Read the model definition and answer for the solid it produces. Units are mm, in the model's axes. Coordinates: 2 decimals unless noted, no trailing zeros. Write each loop counter-clockwise with the first axis right and the second up, starting at its lowest first coordinate (ties: lowest second). Pieces come first, ordered by that corner, then holes. Notation, with made-up numbers: (22, 53.5) -> (28, 53.5) arc R11 ccw to (28, 64.5) -> close; hole circle Ø10 at (19, -32). An arc over 180 degrees is marked (long way). Answer as a JSON object with one key per item and string values. Group by question number.
(1) Find section A-A (y = -19.15). Give the vertices of the cut face in (x, z) (3 decimals), then the cut area to 3 significant figures.
(2) Straight lines are drawn through the part: L1, parallel to X at y = -19.15, z = 1.5 (3 decimals); L2, parallel to Y at x = -14.5, z = 2.9; L3, parallel to X at y = -18, z = 1.85. For each, find the intervals that lie inside material, in ascending order.
(3) Find section D-D (x = -10.15). Give the vertices of the cut face in (y, z) (3 decimals), then the cut area to 3 significant figures.
(4) For a pull along Y with two mould halves and no side action, classify faces 1 (the face through (16.475, -7.375, 1.362)), 2 (the face through (-21.15, 0, 2)), 3 (the face through (0, 28, 2)), 4 (the face through (0, -28, 2)) as +Y half, -Y half, draft (parallel to the pull), parting line (faces both ways), or undercut.
(5) Find section C-C (y = 13). Give the vertices of the cut face in (x, z) (3 decimals), then the cut area to 3 significant figures.
(6) Find section B-B (x = 0). Give the vertices of the cut face in (y, z) (3 decimals), then the cut area to 3 significant figures.
Autodesk Inventor part; units mm, degrees
ref_plane "YZ Plane" through (0, 0, 0) normal (1, 0, 0) x (0, 1, 0)
ref_plane "XZ Plane" through (0, 0, 0) normal (0, 1, 0) x (-1, 0, 0)
ref_plane "XY Plane" through (0, 0, 0) normal (0, 0, 1) x (1, 0, 0)
sketch "Sketch1" plane through (0, 0, 0) normal (0, 0, 1) x (1, 0, 0)
  line L0 (-21.15, 28) -> (21.15, 28)
  line L1 (21.15, 28) -> (21.15, -28)
  line L2 (21.15, -28) -> (-21.15, -28)
  line L3 (-21.15, -28) -> (-21.15, 28)
  point P0 (0, 0)
  dimension "d0" = 56
  dimension "d1" = 42.3
  dimension "d2" = 21.15
  dimension "d3" = 28
  dimension "d44" = 21.15
extrude "Extrusion1" add sketch "Sketch1" along normal blind 3.175
sketch "Sketch2" plane through (0, 0, 3.175) normal (0, 0, 1) x (1, 0, 0)
  circle A0 centre (-15.499, 22.359) radius 1.5875
  circle A1 centre (15.499, 22.359) radius 1.5875
  line L0 (21.15, 28) -> (-21.15, 28)
  line L1 (-21.15, 28) -> (-21.15, -28)
  line L2 (21.15, -28) -> (21.15, 28)
  circle A2 centre (-15.509, -8.635) radius 1.5875
  circle A3 centre (15.509, -8.635) radius 1.5875
  point P0 (0, 0)
  dimension "d6" = 3.175
  dimension "d7" = 5.641
  dimension "d8" = 5.641
  dimension "d9" = 5.651
  dimension "d10" = 5.651
  dimension "d11" = 3.175
  dimension "d45" = 3.175
  dimension "d46" = 3.175
  dimension "d47" = 5.641
  dimension "d48" = 5.641
  dimension "d49" = 36.635
  dimension "d50" = 36.635
hole "Hole1" at (-15.499, 22.359, 3.175) at (15.499, 22.359, 3.175) at (-15.509, -8.635, 3.175) at (15.509, -8.635, 3.175) direction (0, 0, -1) diameter 3.175 end through all countersink diameter 4 countersink angle 90
sketch "Sketch3" plane through (0, 0, 3.175) normal (0, 0, 1) x (1, 0, 0)
  circle A0 centre (-10.15, -19.15) radius 3.175
  circle A1 centre (10.15, -19.15) radius 3.175
  line L0 (-21.15, -28) -> (21.15, -28)
  line L1 (21.15, -28) -> (21.15, 28)
  line L2 (-21.15, 28) -> (-21.15, -28)
  line L3 (21.15, 28) -> (-21.15, 28)
  point P0 (0, 0)
  dimension "d19" = 6.35
  dimension "d20" = 6.35
  dimension "d22" = 11
  dimension "d23" = 11
  dimension "d25" = 47.15
  dimension "d26" = 47.15
hole "Hole2" at (-10.15, -19.15, 3.175) at (10.15, -19.15, 3.175) direction (0, 0, -1) diameter 6.35 end through all
sketch "Sketch5" plane through (0, 0, 0) normal (0, 0, -1) x (-1, 0, 0)
  circle A0 centre (0, 6.756) radius 11.5
  line L0 (21.15, 28) -> (-21.15, 28)
  line L1 (21.15, -28) -> (21.15, 28)
  point P0 (0, 0)
  dimension "d39" = 23
  dimension "d40" = 21.244
  dimension "d41" = 21.15
extrude "Extrusion3" cut sketch "Sketch5" against normal through all
properties part number "MOTOR MOUNT"
Results below:
{
 "1": {"outline": "(-21.15, 0) -> (-13.325, 0) -> (-13.325, 3.175) -> (-21.15, 3.175) -> close; (-6.975, 0) -> (6.975, 0) -> (6.975, 3.175) -> (-6.975, 3.175) -> close; (13.325, 0) -> (21.15, 0) -> (21.15, 3.175) -> (13.325, 3.175) -> close", "area": "94.0 mm2"},
 "2": {"L1": "x = -21.15 to -13.325, -6.975 to 6.975, 13.325 to 21.15", "L2": "y = -28 to -10.03, -7.24 to 20.95, 23.77 to 28", "L3": "x = -21.15 to -13.11, -7.19 to 7.19, 13.11 to 21.15"},
 "3": {"outline": "(-28, 0) -> (-22.325, 0) -> (-22.325, 3.175) -> (-28, 3.175) -> close; (-15.975, 0) -> (1.35, 0) -> (1.35, 3.175) -> (-15.975, 3.175) -> close; (12.162, 0) -> (28, 0) -> (28, 3.175) -> (12.162, 3.175) -> close", "area": "123 mm2"},
 "4": {"face 1": "undercut", "face 2": "draft", "face 3": "+Y half", "face 4": "-Y half"},
 "5": {"outline": "(-21.15, 0) -> (-9.657, 0) -> (-9.657, 3.175) -> (-21.15, 3.175) -> close; (9.657, 0) -> (21.15, 0) -> (21.15, 3.175) -> (9.657, 3.175) -> close", "area": "73.0 mm2"},
 "6": {"outline": "(-28, 0) -> (-4.744, 0) -> (-4.744, 3.175) -> (-28, 3.175) -> close; (18.256, 0) -> (28, 0) -> (28, 3.175) -> (18.256, 3.175) -> close", "area": "105 mm2"}
}
